The model under review builds one solid part; all positions refer to its coordinate system, in mm. A direction names the side the tool comes from. Round coordinates to 2 decimals unless told otherwise and drop trailing zeros. Write each loop counter-clockwise with the first axis right and the second up, starting at its lowest first coordinate (ties: lowest second). Pieces come first, ordered by that corner, then holes. Notation, with made-up numbers: (-3, -0.75) - (40, -0.75) arc R22 ccw to (40, 23.25) - close; hole circle Ø1 at (-18, 42.25). An arc over 180 degrees is marked (long way). Return JSON: item names as keys, results as strings.
from build123d import *

# Parameters (mm, degrees)
F1_DEPTH  = 70
F0_W      = 100
F0_H      = 100
F2_DEPTH  = 130
F3_R      = 50
F4_SIZE   = 60
F0_W_2    = 10
F0_H_2    = 25
F5_DEPTH  = 60
F0_W_3    = 9
F0_H_3    = 20
F6_DEPTH  = 25
F7_DEPTH  = 40
F9_R      = 4
F10_DEPTH = 21
F11_DEPTH = 36.4


with BuildPart() as f1:
    # F0 (on Top) → F1 (new body)
    with BuildSketch(Plane.XY):
        Polygon((-10, -100), (0, -100), (0, 0), (100, 0), (100, 100), (-100, 100), (-100, -100), (-80, -100), (-70, -100), (-70, -75), (-70, -40), (-10, -40), (-10, -75), align=None)
    extrude(amount=F1_DEPTH)

    # F0 (on Top) → F2 (join)
    with BuildSketch(Plane.XY):
        with Locations((50, -50)):
            Rectangle(F0_W, F0_H)
    extrude(amount=F2_DEPTH)

    # F3
    f3_edges = [f1.edges().sort_by_distance(p)[0] for p in [
        (50, 0, 130),
    ]]
    fillet(f3_edges, radius=F3_R)

    # F4
    f4_edges = [f1.edges().sort_by_distance(p)[0] for p in [
        (-85, -100, 70),
        (-5, -100, 70),
    ]]
    chamfer(f4_edges, length=F4_SIZE)

    # F0 (on Top) → F5 (join)
    with BuildSketch(Plane.XY):
        with Locations((-65, -87.5)):
            Rectangle(F0_W_2, F0_H_2)
        with Locations((-15, -87.5)):
            Rectangle(F0_W_2, F0_H_2)
    extrude(amount=F5_DEPTH)

    # F0 (on Top) → F6 (join)
    with BuildSketch(Plane.XY):
        Polygon((-60, -100), (-20, -100), (-20, -75), (-10, -75), (-10, -40), (-70, -40), (-70, -75), (-60, -75), align=None)
        with Locations((-55.5, -60)):
            Rectangle(F0_W_3, F0_H_3, mode=Mode.SUBTRACT)
        with Locations((-24.5, -60)):
            Rectangle(F0_W_3, F0_H_3, mode=Mode.SUBTRACT)
    extrude(amount=F6_DEPTH)

    # F0 (on Top) → F7 (join)
    with BuildSketch(Plane.XY):
        with Locations((-24.5, -60)):
            Rectangle(F0_W_3, F0_H_3)
        with Locations((-55.5, -60)):
            Rectangle(F0_W_3, F0_H_3)
    extrude(amount=F7_DEPTH)

    # F9 (on offset) → F10 (cut, symmetric)
    with BuildSketch(Plane.YZ.offset(-45)):
        with Locations((-60, 34)):
            Circle(F9_R)
    extrude(amount=F10_DEPTH, both=True, mode=Mode.SUBTRACT)

    # F9 (on offset) → F11 (cut, symmetric)
    with BuildSketch(Plane.YZ.offset(-45)):
        with Locations((-87.799012661, 50)):
            Circle(F9_R)
    extrude(amount=F11_DEPTH, both=True, mode=Mode.SUBTRACT)


solid = f1.part
(1) Mouldability with a two-part tool opening along Z and no side actions: class faces 4 (the flat face through (-85, -70, 40)), 5 (the flat face through (-10, -90, 40)), 6 (the cylindrical face through (-26.465, -56.185, 35.201)) as released by +Z, released by -Z, zero draft, split by the parting line, or undercut.
Filled in:
{"face 4": "released by +Z", "face 5": "zero draft", "face 6": "undercut"}
(2) Add section B-B (z = 50). Write out the cut boundary in (x, y).
Filled in:
{"outline": "(-100, -60) - (-70, -60) - (-70, -40) - (-10, -40) - (-10, -60) - (0, -60) - (0, -100) - (100, -100) - (100, 100) - (-100, 100) - close; (-70, -100) - (-60, -100) - (-60, -91.8) - (-70, -91.8) - close; (-70, -83.8) - (-60, -83.8) - (-60, -75) - (-70, -75) - close; (-20, -100) - (-10, -100) - (-10, -91.8) - (-20, -91.8) - close; (-20, -83.8) - (-10, -83.8) - (-10, -75) - (-20, -75) - close"}
(3) Add section D-D (x = -12.5). Write out the cut boundary in (y, z), plus the area to 3 significant figures.
Filled in:
{"outline": "(-100, 0) - (100, 0) - (100, 70) - (-40, 70) - (-40, 25) - (-75, 25) - (-75, 60) - (-100, 60) - close; hole circle Ø8 at (-87.8, 50)", "area": "12,100 mm2"}
(4) Add section C-C (x = 48). Write out the cut boundary in (y, z).
Filled in:
{"outline": "(-100, 0) - (100, 0) - (100, 70) - (0, 70) - (0, 80) arc R50 ccw to (-50, 130) - (-100, 130) - close"}
(5) For faces 1 (the flat face through (-56, -60, 40)), 2 (the flat face through (-24, -60, 34)), 3 (the flat face through (-65, -87, 60)), list the 3-axis set-ups (+Z, -Z, +X, -X, +Y, -Y) from which the entire face can be reached by the end or side of a thin tool; tool diameter is ignored.
Filled in:
{"face 1": "+Z, -Y", "face 2": "none", "face 3": "+Z, -X, -Y"}
(6) Wall thickness on line 1 (Z direction, x = -54.5, y = -60); line 2 (Z direction, x = -40, y = 36); line 3 (Y direction, x = -17, z = 52): over which ranges is each line inside the solid? List them lowest first.
Filled in:
{"line 1": "z = 0 to 30, 38 to 40", "line 2": "z = 0 to 70", "line 3": "y = -100 to -91.26, -84.33 to -75, -40 to 100"}
(7) Add section A-A (y = -60). Write out the cut boundary in (x, z).
Filled in:
{"outline": "(-100, 0) - (100, 0) - (100, 130) - (0, 130) - (0, 50) - (-10, 50) - (-10, 25) - (-20, 25) - (-20, 40) - (-29, 40) - (-29, 38) - (-24, 38) - (-24, 30) - (-29, 30) - (-29, 25) - (-51, 25) - (-51, 30) - (-60, 30) - (-60, 25) - (-70, 25) - (-70, 50) - (-100, 50) - close; (-60, 38) - (-51, 38) - (-51, 40) - (-60, 40) - close"}
(8) Clearance check with flat-ended pins moving along their axes: pin 1 Ø7 at (x, z) = (-26.5, 34.5) entering from -Y; pin 2 Ø4.5 at (x, y) = (-54, -64) entering from +Z; pin 3 Ø1 at (x, z) = (37, 97) entering from +Y. State where each tip first meets the part, or that it passes through.
Filled in:
{"pin 1": "stops at y = -70", "pin 2": "stops at z = 40", "pin 3": "stops at y = -2.8"}
